Source: three-view drawing plus pictorial views. Frame: mm from the lowest corner of the part. A direction names the side the tool comes from. Give positions to 0.01 mm unless a question says otherwise; leave off trailing zeros. Write each loop counter-clockwise with the first axis right and the second up, starting at its lowest first coordinate (ties: lowest second). Pieces come first, ordered by that corner, then holes.
Q1. Line query: L1, parallel to Y at x = 12, z = 2; L2, parallel to Z at x = 10.25, y = 9. Output: solid intervals per line, ascending.
Q2. Pin query (flat end, axial travel): pin 1 (12 mm diameter, centred on x = 11, y = 16, fed in from -Z); pin 2 (6 mm diameter, centred on y = 13, z = 13.5, fed in from -X); pin 3 (1.5 mm diameter, centred on y = 11.5, z = 6.5, fed in from -X). Return the tip coordinate at first contact, or that it passes through.
Q3. Cut plane B-B on x = 16.25. Return the cut outline in (y, z).
Q4. Cut plane C-C on z = 18.5. Return the cut outline in (x, y).
Q5. Cut plane A-A on y = 21. Return the cut outline in (x, z).
Q6. Reachability of the marked faces 1 and 2 from +Z, -Z, +X, -X, +Y, -Y: full face, straight path, thin tool, end or side. Return the list, or none.
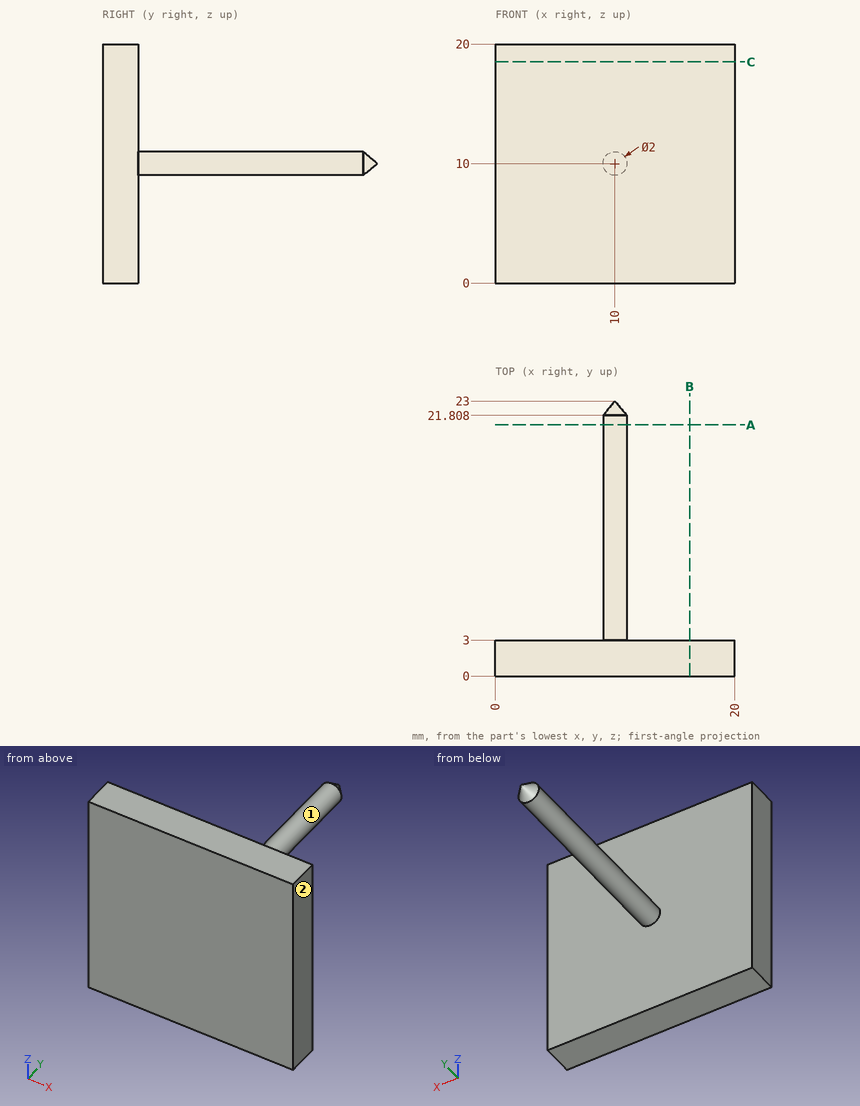
Data:
1. L1: y = 0 to 3
1. L2: z = 9.03 to 10.97
2. pin 1: stops at z = 9
2. pin 2: stops at x = 9.13
2. pin 3: passes through
3. outline: (0, 0) - (3, 0) - (3, 20) - (0, 20) - close
4. outline: (0, 0) - (20, 0) - (20, 3) - (0, 3) - close
5. outline: circle Ø2 at (10, 10)
6. face 1: +Y
6. face 2: +Z, -Z, +X, +Y, -Y
